Work out the finished part from the listing and answer in its coordinate system (mm). A direction names the side the tool comes from. Coordinates: 2 decimals unless noted, no trailing zeros. Write each loop counter-clockwise with the first axis right and the second up, starting at its lowest first coordinate (ties: lowest second). Pieces come first, ordered by that corner, then holes. Notation, with made-up numbers: (14, -15) - (32, -15) arc R31 ccw to (32, 23) - close; hole circle Ø1 at (-22, 80). An arc over 180 degrees is marked (long way). Use CSV: the item, a comma, the result in double quotes. Start each with the question number.
from build123d import *

# Parameters (mm, degrees)
SKETCH1_R               = 10.16
BOSS_EXTRUDE1_DEPTH     = 12.7
SKETCH2_R               = 14.2875
CUT_EXTRUDE1_DEPTH      = 7.9375
CUT_EXTRUDE2_DEPTH      = 5
CUT_EXTRUDE3_START      = 12.7
CUT_EXTRUDE3_DEPTH      = 2
CUT_EXTRUDE4_DEPTH      = 22
CUT_EXTRUDE4_DEPTH_BACK = 12
SKETCH6_R               = 27.94
BOSS_EXTRUDE2_DEPTH     = 32


with BuildPart() as part:
    # Sketch1 → Boss-Extrude1 (new body)
    with BuildSketch(Plane(origin=(0, 0, 0), x_dir=(1, 0, 0), z_dir=(0, 1, 0))):
        with BuildLine():
            Line((-42.9, 47.5), (42.9, 47.5))
            Line((42.9, 47.5), (101.65500633, 36.904754311))
            ThreePointArc((101.65500633, 36.904754311), (132.5, 0), (101.65500633, -36.904754311))
            Line((101.65500633, -36.904754311), (42.9, -47.5))
            Line((42.9, -47.5), (-42.9, -47.5))
            Line((-42.9, -47.5), (-95, -20))
            ThreePointArc((-95, -20), (-115, 0), (-95, 20))
            Line((-95, 20), (-42.9, 47.5))
        make_face()
        with Locations(Location((-95, 0, 0), (0, 0, 270))):
            Circle(SKETCH1_R, mode=Mode.SUBTRACT)
        with Locations(Location((95, 0, 0), (0, 0, 270))):
            Circle(SKETCH1_R, mode=Mode.SUBTRACT)
        with BuildLine():
            Line((-42.3, 37.85), (-27.3, 37.85))
            ThreePointArc((-27.3, 37.85), (-24.25, 34.8), (-27.3, 31.75))
            Line((-27.3, 31.75), (-42.3, 31.75))
            ThreePointArc((-42.3, 31.75), (-45.35, 34.8), (-42.3, 37.85))
        make_face(mode=Mode.SUBTRACT)
        with BuildLine():
            Line((42.3, 31.75), (27.3, 31.75))
            ThreePointArc((27.3, 31.75), (24.25, 34.8), (27.3, 37.85))
            Line((27.3, 37.85), (42.3, 37.85))
            ThreePointArc((42.3, 37.85), (45.35, 34.8), (42.3, 31.75))
        make_face(mode=Mode.SUBTRACT)
        with BuildLine():
            Line((42.3, -37.85), (27.3, -37.85))
            ThreePointArc((27.3, -37.85), (24.25, -34.8), (27.3, -31.75))
            Line((27.3, -31.75), (42.3, -31.75))
            ThreePointArc((42.3, -31.75), (45.35, -34.8), (42.3, -37.85))
        make_face(mode=Mode.SUBTRACT)
        with BuildLine():
            Line((-42.3, -31.75), (-27.3, -31.75))
            ThreePointArc((-27.3, -31.75), (-24.25, -34.8), (-27.3, -37.85))
            Line((-27.3, -37.85), (-42.3, -37.85))
            ThreePointArc((-42.3, -37.85), (-45.35, -34.8), (-42.3, -31.75))
        make_face(mode=Mode.SUBTRACT)
        with BuildLine():
            Line((-8, 7.5), (8, 7.5))
            ThreePointArc((8, 7.5), (15.5, 0), (8, -7.5))
            Line((8, -7.5), (-8, -7.5))
            ThreePointArc((-8, -7.5), (-15.5, 0), (-8, 7.5))
        make_face(mode=Mode.SUBTRACT)
    extrude(amount=BOSS_EXTRUDE1_DEPTH)

    # Sketch2 → Cut-Extrude1 (cut)
    with BuildSketch(Plane(origin=(0, 0, 0), x_dir=(1, 0, 0), z_dir=(0, 1, 0))):
        with Locations(Location((-95, 0, 0), (0, 0, 270))):
            Circle(SKETCH2_R)
        with Locations(Location((95, 0, 0), (0, 0, 270))):
            Circle(SKETCH2_R)
    extrude(amount=CUT_EXTRUDE1_DEPTH, mode=Mode.SUBTRACT)

    # Sketch3 → Cut-Extrude2 (cut)
    with BuildSketch(Plane(origin=(0, 0, 0), x_dir=(1, 0, 0), z_dir=(0, 1, 0))):
        with BuildLine():
            Line((-40.8, -40.05), (-28.8, -40.05))
            ThreePointArc((-28.8, -40.05), (-23.55, -34.8), (-28.8, -29.55))
            Line((-28.8, -29.55), (-40.8, -29.55))
            ThreePointArc((-40.8, -29.55), (-46.05, -34.8), (-40.8, -40.05))
        make_face()
        with BuildLine():
            Line((40.8, -29.55), (28.8, -29.55))
            ThreePointArc((28.8, -29.55), (23.55, -34.8), (28.8, -40.05))
            Line((28.8, -40.05), (40.8, -40.05))
            ThreePointArc((40.8, -40.05), (46.05, -34.8), (40.8, -29.55))
        make_face()
        with BuildLine():
            Line((40.8, 40.05), (28.8, 40.05))
            ThreePointArc((28.8, 40.05), (23.55, 34.8), (28.8, 29.55))
            Line((28.8, 29.55), (40.8, 29.55))
            ThreePointArc((40.8, 29.55), (46.05, 34.8), (40.8, 40.05))
        make_face()
        with BuildLine():
            ThreePointArc((-28.8, 29.55), (-23.55, 34.8), (-28.8, 40.05))
            Line((-28.8, 40.05), (-40.8, 40.05))
            ThreePointArc((-40.8, 40.05), (-46.05, 34.8), (-40.8, 29.55))
            Line((-40.8, 29.55), (-28.8, 29.55))
        make_face()
    extrude(amount=CUT_EXTRUDE2_DEPTH, mode=Mode.SUBTRACT)

    # Sketch4 → Cut-Extrude3 (cut)
    with BuildSketch(Plane(origin=(0, 0, 0), x_dir=(1, 0, 0), z_dir=(0, 1, 0)).offset(CUT_EXTRUDE3_START)):
        with BuildLine():
            Line((-5, 34.8), (5, 34.8))
            ThreePointArc((5, 34.8), (39.8, 0), (5, -34.8))
            Line((5, -34.8), (-5, -34.8))
            ThreePointArc((-5, -34.8), (-39.8, 0), (-5, 34.8))
        make_face()
    extrude(amount=-CUT_EXTRUDE3_DEPTH, mode=Mode.SUBTRACT)

    # Sketch5 → Cut-Extrude4 (cut, two sides: drawn at the far end of the back side and taken through both)
    with BuildSketch(Plane(origin=(0, 0, 0), x_dir=(1, 0, 0), z_dir=(0, 1, 0)).offset(-CUT_EXTRUDE4_DEPTH_BACK)):
        with BuildLine():
            Line((-7.5, 20.32), (7.5, 20.32))
            ThreePointArc((7.5, 20.32), (27.82, 0), (7.5, -20.32))
            Line((7.5, -20.32), (-7.5, -20.32))
            ThreePointArc((-7.5, -20.32), (-27.82, 0), (-7.5, 20.32))
        make_face()
    extrude(amount=CUT_EXTRUDE4_DEPTH + CUT_EXTRUDE4_DEPTH_BACK, mode=Mode.SUBTRACT)

    # Sketch6 → Boss-Extrude2 (add)
    with BuildSketch(Plane(origin=(0, 0, 0), x_dir=(1, 0, 0), z_dir=(0, 1, 0))):
        with Locations(Location((0, 0, 0), (0, 0, 270))):
            Circle(SKETCH6_R)
    extrude(amount=-BOSS_EXTRUDE2_DEPTH)


solid = part.part
Item 1: A cutting plane is placed at B-B (y = -26). Determine the outline of the cut face in (x, z).
Item 2: A cutting plane is placed at C-C (x = 69). Determine the outline of the cut face in (y, z).
Item 3: Straight lines are drawn through the part: probe 1 along X at (y, z) = (5, 0); probe 2 along X at (y, z) = (9.95, 0); probe 3 along Z at (x, y) = (-95, 10). For each, find the intervals that lie inside material, in ascending order. Write a range as [from, to].
Item 4: Each of these flat-tipped pins is pushed along its axis until it touches: pin 1 (3 mm diameter, centred on x = -38.5, z = -33, fed in from -Y); pin 2 (8 mm diameter, centred on y = 3.5, z = -32, fed in from -X); pin 3 (2 mm diameter, centred on y = 7.5, z = -8, fed in from +X). Where does it stop, or does it pass through?
Item 5: Determine the mould class of faces 6 (the face through (27.7, -15.78, -3.64)), 7 (the face through (1, 6, 47.5)), 8 (the face through (24.25, 8.8, -34.73)) for opening direction X: +X half, -X half, draft (parallel to the pull), parting line (faces both ways), or undercut.
Item 6: A cutting plane is placed at D-D (x = -62). Determine the outline of the cut face in (y, z).
Item 7: A cutting plane is placed at A-A (x = 95). Determine the outline of the cut face in (y, z).
Item 8: Which of the six approach directions +Z, -Z, +X, -X, +Y, -Y give full straight-line access (tool end or side, diameter ignored) to faces 1 (the face through (-27.815, 5.275, 0.447)), 2 (the face through (0, -32, 0)), 3 (the face through (132.493, 6.261, -0.731)), 4 (the face through (35, 9, 37.85)), 5 (the face through (-46.05, 2.46, -34.92))?
Calculated:
1,outline,"circle Ø55.88 at (0, 0)"
2,outline,"(0, -42.79) - (12.7, -42.79) - (12.7, 42.79) - (0, 42.79) - close"
3,probe 1,"x = [-115, -109.29], [-80.71, -27.82], [27.82, 80.71], [109.29, 132.5]"
3,probe 2,"x = [-115, -105.16], [-84.84, -27.82], [27.82, 84.84], [105.16, 132.5]"
3,probe 3,"z = [-20, -10.16], [10.16, 20]"
4,pin 1,"stops at y = 5"
4,pin 2,"stops at x = -79.84"
4,pin 3,"stops at x = 131.84"
5,face 6,"parting line"
5,face 7,"draft"
5,face 8,"undercut"
6,outline,"(0, -37.42) - (12.7, -37.42) - (12.7, 37.42) - (0, 37.42) - close"
7,outline,"(0, -38.1) - (12.7, -38.1) - (12.7, -10.16) - (7.94, -10.16) - (7.94, -14.29) - (0, -14.29) - close; (0, 14.29) - (7.94, 14.29) - (7.94, 10.16) - (12.7, 10.16) - (12.7, 38.1) - (0, 38.1) - close"
8,face 1,"+Y"
8,face 2,"+Z, -Z, +X, -X, -Y"
8,face 3,"+X, +Y, -Y"
8,face 4,"+Y, -Y"
8,face 5,"-Y"
